For this review, take the finished solid that the model builds, in its own axes (mm). A direction names the side the tool comes from. Round coordinates to 2 decimals unless told otherwise and drop trailing zeros. Loops run counter-clockwise (first coordinate to the right, second up) from the corner with the lowest first, then second, coordinate; pieces in that order, holes last.
1. Consider section D-D on z = 15. State how many separate pieces and enclosed holes the cut face has, then the cut area to 3 significant figures.
2. Tool access review of faces 4 (the flat face through (1, 15.7, 13)), 5 (the flat face through (-7.5, 16, 12)), 6 (the flat face through (0, -2, 2.5)): name each direction out of +Z, -Z, +X, -X, +Y, -Y from which nothing blocks a thin tool from reaching the whole face with its end or side.
3. Consider section C-C on x = 19.5. State the section outline as (y, z) points.
4. To check wall thickness, follow line 1 along X through (y, z) = (16, 10); line 2 along Y through (x, z) = (-22.5, 6); line 3 along Z through (x, y) = (0, 16.6). State the ranges of each line that lie inside material, in increasing order.
5. Clearance check with flat-ended pins moving along their axes: pin 1 Ø2.5 at (x, y) = (11.5, 17.5) entering from +Z; pin 2 Ø6 at (x, z) = (0, 15) entering from -Y; pin 3 Ø4 at (x, y) = (-3, 12) entering from +Z. State where each tip first meets the part, or that it passes through.
6. Draft analysis for pull direction Z (two halves, no side actions). For faces 1 (the flat face through (-14, 16, 2.5)), 2 (the flat face through (29, 15.7, 15)), 3 (the flat face through (0, 11.7, 21)), state which applies: released by +Z, released by -Z, zero draft, split by the parting line, or undercut.
7. Consider section A-A on z = 6.5. State the section outline as (x, y) points.
8. Consider section B-B on x = 0. State the section outline as (y, z) points.
from build123d import *

# Parameters (mm, degrees)
F0_W     = 13.25
F0_H     = 4.8
F0_W_2   = 65.5
F0_H_2   = 27
F0_H_3   = 3.2
F1_DEPTH = 2.5
F2_DEPTH = 27.5
F3_DEPTH = 42.5
F4_R     = 1.9
F5_DEPTH = 6.801
F4_R_2   = 4.5
F6_DEPTH = 4
F4_R_3   = 5.5
F7_DEPTH = 30.201
F8_R     = 5
F9_R     = 2


with BuildPart() as f1:
    # F0 (on Top) → F1 (new body)
    with BuildSketch(Plane.XY):
        Polygon((-20.75, 18.5), (-32.75, 18.5), (-32.75, 11.7), (32.75, 11.7), (32.75, 18.5), (20.75, 18.5), (20.75, 13.7), (7.5, 13.7), (7.5, 18.5), (-7.5, 18.5), (-7.5, 13.7), (-20.75, 13.7), align=None)
        with Locations((-14.125, 16.1)):
            Rectangle(F0_W, F0_H)
        with Locations((0, -1.8)):
            Rectangle(F0_W_2, F0_H_2)
        with Locations((0, -16.9)):
            Rectangle(F0_W_2, F0_H_3)
        with Locations((14.125, 16.1)):
            Rectangle(F0_W, F0_H)
    extrude(amount=F1_DEPTH)

    # F0 (on Top) → F2 (join)
    with BuildSketch(Plane.XY):
        Polygon((-20.75, 18.5), (-32.75, 18.5), (-32.75, 11.7), (32.75, 11.7), (32.75, 18.5), (20.75, 18.5), (20.75, 13.7), (7.5, 13.7), (7.5, 18.5), (-7.5, 18.5), (-7.5, 13.7), (-20.75, 13.7), align=None)
    extrude(amount=F2_DEPTH)

    # F0 (on Top) → F3 (join)
    with BuildSketch(Plane.XY):
        with Locations((0, -16.9)):
            Rectangle(F0_W_2, F0_H_3)
    extrude(amount=F3_DEPTH)

    # F4 (on face) → F5 (cut, through all)
    with BuildSketch(Plane.XZ.offset(-11.7)):
        with Locations((-26.75, 15)):
            Circle(F4_R)
        with Locations((0, 15)):
            Circle(F4_R)
        with Locations((26.75, 15)):
            Circle(F4_R)
    extrude(amount=-F5_DEPTH, mode=Mode.SUBTRACT)

    # F4 (on face) → F6 (cut)
    with BuildSketch(Plane.XZ.offset(-11.7)):
        with BuildLine():
            ThreePointArc((-31.25, 15), (-26.75, 10.5), (-22.25, 15))
            ThreePointArc((-22.25, 15), (-26.75, 19.5), (-31.25, 15))
        make_face()
        with Locations((-26.75, 15)):
            Circle(F4_R, mode=Mode.SUBTRACT)
        with Locations((26.75, 15)):
            Circle(F4_R_2)
        with Locations((26.75, 15)):
            Circle(F4_R, mode=Mode.SUBTRACT)
        with Locations((0, 15)):
            Circle(F4_R_2)
        with Locations((0, 15)):
            Circle(F4_R, mode=Mode.SUBTRACT)
    extrude(amount=-F6_DEPTH, mode=Mode.SUBTRACT)

    # F4 (on face) → F7 (cut, through all)
    with BuildSketch(Plane.XZ.offset(-11.7)):
        with Locations((25.75, 15)):
            Circle(F4_R_3)
        with Locations((26.75, 15)):
            Circle(F4_R_2, mode=Mode.SUBTRACT)
        with Locations((0, 15)):
            Circle(F4_R_3)
        with Locations((0, 15)):
            Circle(F4_R_2, mode=Mode.SUBTRACT)
        with BuildLine():
            ThreePointArc((-20.25, 15), (-25.75, 20.5), (-31.25, 15))
            ThreePointArc((-31.25, 15), (-25.75, 9.5), (-20.25, 15))
        make_face()
        with BuildLine():
            ThreePointArc((-31.25, 15), (-26.75, 19.5), (-22.25, 15))
            ThreePointArc((-22.25, 15), (-26.75, 10.5), (-31.25, 15))
        make_face(mode=Mode.SUBTRACT)
        with Locations((26.75, 15)):
            Circle(F4_R_2)
        with Locations((26.75, 15)):
            Circle(F4_R, mode=Mode.SUBTRACT)
        with Locations((0, 15)):
            Circle(F4_R_2)
        with Locations((0, 15)):
            Circle(F4_R, mode=Mode.SUBTRACT)
        with BuildLine():
            ThreePointArc((-31.25, 15), (-26.75, 10.5), (-22.25, 15))
            ThreePointArc((-22.25, 15), (-26.75, 19.5), (-31.25, 15))
        make_face()
        with Locations((-26.75, 15)):
            Circle(F4_R, mode=Mode.SUBTRACT)
        with Locations((26.75, 15)):
            Circle(F4_R)
        with Locations((0, 15)):
            Circle(F4_R)
        with Locations((-26.75, 15)):
            Circle(F4_R)
    extrude(amount=F7_DEPTH, mode=Mode.SUBTRACT)

    # F8
    f8_edges = [f1.edges().sort_by_distance(p)[0] for p in [
        (-32.75, 15.1, 27.5),
        (32.75, 15.1, 27.5),
        (20.75, 16.1, 27.5),
        (7.5, 16.1, 27.5),
        (-7.5, 16.1, 27.5),
        (-20.75, 16.1, 27.5),
        (32.75, -16.9, 42.5),
        (-32.75, -16.9, 42.5),
    ]]
    fillet(f8_edges, radius=F8_R)

    # F9
    f9_edges = [f1.edges().sort_by_distance(p)[0] for p in [
        (0, -15.3, 2.5),
        (0, 11.7, 2.5),
    ]]
    fillet(f9_edges, radius=F9_R)


solid = f1.part
Resolved:
1. separate pieces: 8
1. enclosed holes: 0
1. area: 282 mm2
2. face 4: -Y
2. face 5: +Z, +Y
2. face 6: +Z, +X, -X
3. outline: (-18.5, 0) - (18.5, 0) - (18.5, 2.5) - (13.7, 2.5) - (13.7, 27.5) - (11.7, 27.5) - (11.7, 4.5) arc R2 cw to (9.7, 2.5) - (-13.3, 2.5) arc R2 cw to (-15.3, 4.5) - (-15.3, 42.5) - (-18.5, 42.5) - close
4. line 1: x = -32.75 to -20.75, -7.5 to 7.5, 20.75 to 32.75
4. line 2: y = -18.5 to -15.3, 11.7 to 18.5
4. line 3: z = 0 to 13.1, 16.9 to 27.5
5. pin 1: stops at z = 2.5
5. pin 2: stops at y = 15.7
5. pin 3: stops at z = 27.5
6. face 1: released by +Z
6. face 2: undercut
6. face 3: zero draft
7. outline: (-32.75, -18.5) - (32.75, -18.5) - (32.75, -15.3) - (-32.75, -15.3) - close; (-32.75, 11.7) - (32.75, 11.7) - (32.75, 18.5) - (20.75, 18.5) - (20.75, 13.7) - (7.5, 13.7) - (7.5, 18.5) - (-7.5, 18.5) - (-7.5, 13.7) - (-20.75, 13.7) - (-20.75, 18.5) - (-32.75, 18.5) - close
8. outline: (-18.5, 0) - (18.5, 0) - (18.5, 13.1) - (15.7, 13.1) - (15.7, 10.5) - (11.7, 10.5) - (11.7, 4.5) arc R2 cw to (9.7, 2.5) - (-13.3, 2.5) arc R2 cw to (-15.3, 4.5) - (-15.3, 9.5) - (-18.5, 9.5) - close; (-18.5, 20.5) - (-15.3, 20.5) - (-15.3, 42.5) - (-18.5, 42.5) - close; (11.7, 19.5) - (15.7, 19.5) - (15.7, 16.9) - (18.5, 16.9) - (18.5, 27.5) - (11.7, 27.5) - close
